from build123d import *

# Parameters (mm, degrees)
SKETCH_1_W                 = 240
SKETCH_1_H                 = 100
EXTRUDE_1_DEPTH            = 6
SKETCH_2_R                 = 1.55
CUT_EXTRUDE_1_DEPTH        = 261.069221555
SKETCH_3_W                 = 60
SKETCH_3_H                 = 15
CUT_EXTRUDE_2_DEPTH        = 261.069221555
SKETCH_4_W                 = 30
SKETCH_4_H                 = 60
CUT_EXTRUDE_3_DEPTH        = 261.069221555
SKETCH_5_R                 = 3
CUT_EXTRUDE_4_DEPTH        = 3
EXTRUDE_2_DEPTH            = 240
EXTRUDE_3_DEPTH            = 5
PATTERN_LINEAR_5_COUNT     = 6
PATTERN_LINEAR_5_PITCH     = 20
PATTERN_LINEAR_5_COL_COUNT = 6
PATTERN_LINEAR_5_COL_PITCH = 20
FILLET_5_R                 = 5
CHAMFER_1_SIZE             = 3
CUT_EXTRUDE_7_DEPTH        = 261.069221555


with BuildPart() as part:
    # 草图1 → 凸台-拉伸1 (new body)
    with BuildSketch(Plane(origin=(0, 0, 0), x_dir=(0, 0, -1), z_dir=(1, 0, 0))):
        with Locations((120, -50)):
            Rectangle(SKETCH_1_W, SKETCH_1_H)
    extrude(amount=EXTRUDE_1_DEPTH)

    # 草图2 → 切除-拉伸1 (cut, through all)
    with BuildSketch(Plane(origin=(6, 0, 0), x_dir=(0, 0, -1), z_dir=(1, 0, 0))):
        with Locations((19.32352941, -54)):
            Circle(SKETCH_2_R)
        with Locations((56.32352941, -80)):
            Circle(SKETCH_2_R)
        with Locations((56.32352941, -54)):
            Circle(SKETCH_2_R)
        with Locations((19.32352941, -80)):
            Circle(SKETCH_2_R)
        with Locations(Location((220.67647059, -80, 0), (0, 0, 180))):
            Circle(SKETCH_2_R)
        with Locations(Location((183.67647059, -54, 0), (0, 0, 180))):
            Circle(SKETCH_2_R)
        with Locations(Location((183.67647059, -80, 0), (0, 0, 180))):
            Circle(SKETCH_2_R)
        with Locations(Location((220.67647059, -54, 0), (0, 0, 180))):
            Circle(SKETCH_2_R)
    extrude(amount=-CUT_EXTRUDE_1_DEPTH, mode=Mode.SUBTRACT)

    # 草图3 → 切除-拉伸2 (cut, through all)
    with BuildSketch(Plane(origin=(6, 0, 0), x_dir=(0, 0, -1), z_dir=(1, 0, 0))):
        with Locations((40, -27.5)):
            Rectangle(SKETCH_3_W, SKETCH_3_H)
        with Locations((200, -27.5)):
            Rectangle(SKETCH_3_W, SKETCH_3_H)
    extrude(amount=-CUT_EXTRUDE_2_DEPTH, mode=Mode.SUBTRACT)

    # 草图4 → 切除-拉伸3 (cut, through all)
    with BuildSketch(Plane(origin=(6, 0, 0), x_dir=(0, 0, -1), z_dir=(1, 0, 0))):
        with Locations((100, -40)):
            Rectangle(SKETCH_4_W, SKETCH_4_H)
        with Locations((140, -40)):
            Rectangle(SKETCH_4_W, SKETCH_4_H)
    extrude(amount=-CUT_EXTRUDE_3_DEPTH, mode=Mode.SUBTRACT)

    # 草图5 → 切除-拉伸4 (cut)
    with BuildSketch(Plane.ZY):
        with Locations((-183.67647059, -80)):
            Circle(SKETCH_5_R)
        with Locations((-220.67647059, -80)):
            Circle(SKETCH_5_R)
        with Locations((-183.67647059, -54)):
            Circle(SKETCH_5_R)
        with Locations((-220.67647059, -54)):
            Circle(SKETCH_5_R)
        with Locations((-45, -80)):
            Circle(SKETCH_5_R)
        with Locations((-19.32352941, -80)):
            Circle(SKETCH_5_R)
        with Locations((-19.32352941, -54)):
            Circle(SKETCH_5_R)
        with Locations((-56.32352941, -54)):
            Circle(SKETCH_5_R)
    extrude(amount=-CUT_EXTRUDE_4_DEPTH, mode=Mode.SUBTRACT)

    # 草图6 → 凸台-拉伸2 (add)
    with BuildSketch(Plane.XY):
        Polygon((6, 0), (0, 0), (0, 10.392304845), align=None)
    extrude(amount=-EXTRUDE_2_DEPTH)

    # 草图7 → 凸台-拉伸3 (add)
    with BuildSketch(Plane.XY.offset(-117.5)):
        Polygon((0, 10.392304845), (0, 15.392304845), (8, 1.535898385), (8, -8), (6, -8), (6, 0), align=None)
    extrude_3 = extrude(amount=-EXTRUDE_3_DEPTH)

    # 阵列(线性)5: 凸台-拉伸3 ×6
    with Locations(*[(0, 0, i * PATTERN_LINEAR_5_PITCH) for i in range(1, PATTERN_LINEAR_5_COUNT)]):
        add(extrude_3)

    # 阵列(线性)5 col: 凸台-拉伸3 ×6
    with Locations(*[(0, 0, -i * PATTERN_LINEAR_5_COL_PITCH) for i in range(1, PATTERN_LINEAR_5_COL_COUNT)]):
        add(extrude_3)

    # 圆角5
    fillet_5_edges = [part.edges().sort_by_distance(p)[0] for p in [
        (8, 1.535898385, -120),
        (8, 1.535898385, -140),
        (8, 1.535898385, -160),
        (8, 1.535898385, -180),
        (8, 1.535898385, -200),
        (8, 1.535898385, -220),
        (8, 1.535898385, -100),
        (8, 1.535898385, -80),
        (8, 1.535898385, -60),
        (8, 1.535898385, -40),
        (8, 1.535898385, -20),
    ]]
    fillet(fillet_5_edges, radius=FILLET_5_R)

    # 倒角1
    chamfer_1_edges = [part.edges().sort_by_distance(p)[0] for p in [
        (3, -35, -10),
        (3, -20, -10),
        (3, -20, -70),
        (3, -35, -70),
        (3, -20, -170),
        (3, -20, -230),
        (3, -35, -230),
        (3, -35, -170),
        (3, -10, -115),
        (3, -70, -115),
        (3, -70, -85),
        (3, -10, -85),
        (3, -10, -125),
        (3, -10, -155),
        (3, -70, -155),
        (3, -70, -125),
    ]]
    chamfer(chamfer_1_edges, length=CHAMFER_1_SIZE)

    # 草图8 → 切除-拉伸7 (cut, through all)
    with BuildSketch(Plane(origin=(6, 0, 0), x_dir=(0, 0, -1), z_dir=(1, 0, 0))):
        Polygon((85, -100), (85, -83), (88, -80), (152, -80), (155, -83), (155, -100), align=None)
    extrude(amount=-CUT_EXTRUDE_7_DEPTH, mode=Mode.SUBTRACT)


solid = part.part
For this review, take the finished solid that the model builds, in its own axes (mm). A direction names the side the tool comes from. Give positions to 0.01 mm unless a question says otherwise; leave off trailing zeros. Order: outer loops, then holes, each group sorted by start corner. A loop starts at its lowest first (then second) coordinate and runs counter-clockwise, first axis right, second up. Notation, with made-up numbers: (50.25, 50) - (70.25, 50) arc R24 cw to (70.25, 73) - close; hole circle Ø3 at (-20.75, -25). An arc over 180 degrees is marked (long way). Answer as a JSON object with one key per item and string values. Group by question number.
Item 1: Machinability: for faces 4 (the flat face through (3, -100, -197)), 5 (the flat face through (3, -80, -120)), 6 (the flat face through (3, -10, -100)), 7 (the flat face through (8, -4, -60)), 8 (the flat face through (5, 4, -42.5)), which of the approach directions +Z, -Z, +X, -X, +Y, -Y give a long, thin tool a straight path to every point of the face, cutting with its end or side? Answer none if there is none.
Item 2: Draft analysis for pull direction Z (two halves, no side actions). For faces 1 (the flat face through (2.958, 5.269, -69.895)), 2 (the flat face through (5, 4, -182.5)), 3 (the flat face through (3.614, 9.133, -139.965)), state which applies: pulls with the +Z half, pulls with the -Z half, needs draft (parallel to the pull), parting line crosses it, or undercut.
Item 3: Take a section at B-B on x = 1.75. Give the number of separate pieces and of enclosed holes in the cut face, and give its area (3 significant figures).
Item 4: Take a section at A-A on z = -25. Give the boundary of the cut face in (x, y).
Item 5: Take a section at C-C on z = -165.5. Give the boundary of the cut face in (x, y).
Item 6: Clearance check with flat-ended pins moving along their axes: pin 1 Ø5 at (y, z) = (-80, -220.68) entering from -X; pin 2 Ø4 at (x, z) = (3, -127.5) entering from -Y; pin 3 Ø1 at (y, z) = (-87.5, -203.5) entering from +X. State where each tip first meets the part, or that it passes through.
Item 7: Wall thickness on line 1 along Z through (x, y) = (1.25, -23.5); line 2 along Z through (x, y) = (3, -18); line 3 along Z through (x, y) = (2, -86): over which ranges is each line inside the solid? List them lowest first.
Reported:
{
 "1": {"face 4": "+Z, -Z, +X, -X, -Y", "face 5": "+X, -X, -Y", "face 6": "+X, -X", "face 7": "+Z, -Z, +X, +Y, -Y", "face 8": "+X, +Y"},
 "2": {"face 1": "undercut", "face 2": "undercut", "face 3": "needs draft"},
 "3": {"separate pieces": "1", "enclosed holes": "13", "area": "19,100 mm^2"},
 "4": {"outline": "(0, -100) - (6, -100) - (6, -35) - (0, -35) - close; (0, -20) - (6, -20) - (6, 0) - (0, 10.39) - close"},
 "5": {"outline": "(0, -100) - (6, -100) - (6, 0) - (0, 10.39) - close"},
 "6": {"pin 1": "x = 3", "pin 2": "y = -80", "pin 3": "x = 6"},
 "7": {"line 1": "-240 to -230, -170 to -155, -125 to -115, -85 to -70, -10 to 0", "line 2": "-240 to -155, -125 to -115, -85 to 0", "line 3": "-240 to -155, -85 to 0"}
}
